Input: part model. Units: mm. Frame: model coordinates. Face numbers are marked on the shaded views. A direction names the side the tool comes from. Round coordinates to 2 decimals unless told otherwise and drop trailing zeros. Write each loop counter-clockwise with the first axis right and the second up, starting at its lowest first coordinate (ties: lowest second). Pieces come first, ordered by that corner, then holes. Notation, with made-up numbers: (82, 11) -> (139, 11) arc R18 cw to (139, 40) -> close; hole circle Ø10 at (63, -25). An arc over 180 degrees is marked (long way). Write item = value, one per line.
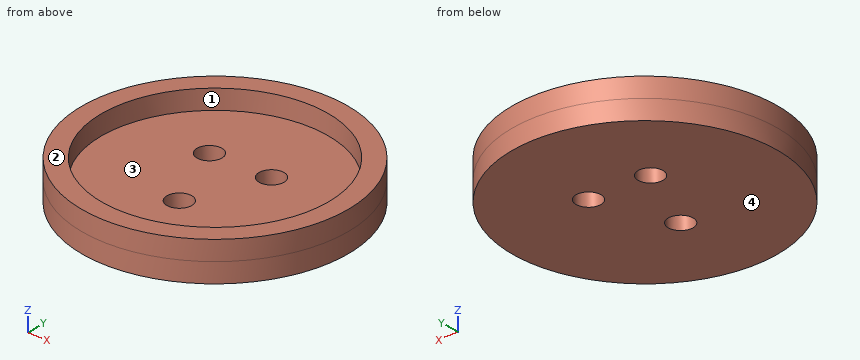
```python
from build123d import *

# Parameters (mm, degrees)
SKETCH1_R      = 24
EXTRUDE1_DEPTH = 4
SKETCH2_R      = 24
EXTRUDE2_DEPTH = 1
SKETCH3_R      = 3.2
EXTRUDE3_DEPTH = 6
SKETCH4_R      = 34
SKETCH4_R_2    = 24
EXTRUDE4_DEPTH = 5
SKETCH5_R      = 34
SKETCH5_R_2    = 29
EXTRUDE5_DEPTH = 5


with BuildPart() as part:
    # Sketch1 → Extrude1 (new body)
    with BuildSketch(Plane.XY):
        Circle(SKETCH1_R)
    extrude(amount=EXTRUDE1_DEPTH)

    # Sketch2 → Extrude2 (add)
    with BuildSketch(Plane.XY.offset(4)):
        Circle(SKETCH2_R)
    extrude(amount=EXTRUDE2_DEPTH)

    # Sketch3 → Extrude3 (cut, through all)
    with BuildSketch(Plane.XY.offset(5)):
        with Locations((-7.9375, 7.9375)):
            Circle(SKETCH3_R)
        with Locations((7.9375, 7.9375)):
            Circle(SKETCH3_R)
        with Locations((0, -11.1125)):
            Circle(SKETCH3_R)
    extrude(amount=-EXTRUDE3_DEPTH, mode=Mode.SUBTRACT)

    # Sketch4 → Extrude4 (add)
    with BuildSketch(Plane(origin=(0, 0, 0), x_dir=(-1, 0, 0), z_dir=(0, 0, -1))):
        Circle(SKETCH4_R)
        Circle(SKETCH4_R_2, mode=Mode.SUBTRACT)
    extrude(amount=-EXTRUDE4_DEPTH)

    # Sketch5 → Extrude5 (add)
    with BuildSketch(Plane.XY.offset(5)):
        Circle(SKETCH5_R)
        Circle(SKETCH5_R_2, mode=Mode.SUBTRACT)
    extrude(amount=EXTRUDE5_DEPTH)


solid = part.part
```
1) Cut plane A-A (x = 0). Return the cut outline in (y, z).
Solutions:
outline = (-34, 0) -> (-14.31, 0) -> (-14.31, 5) -> (-29, 5) -> (-29, 10) -> (-34, 10) -> close; (-7.91, 0) -> (34, 0) -> (34, 10) -> (29, 10) -> (29, 5) -> (-7.91, 5) -> close
2) Draft query along Y for the marked faces 3 and 4. Return one class per face: +Y half, -Y half, draft (parallel to the pull), parting line (faces both ways), or undercut.
Solutions:
face_3 = undercut
face_4 = draft
3) First-contact query: P1, Ø17.5, axis at x = 4.5, y = -2, coming from the +Z side; P2, Ø6, axis at x = 7.94, y = 7.94, coming from the +Z side; P3, Ø6, axis at x = 18, y = 10.5, coming from the -Z side; P4, Ø1.5, axis at y = 3, z = 5.5, coming from the +X side. Flat tips, straight axial feed; report the tip coordinate or a pass-through.
Solutions:
P1 = 5
P2 = through
P3 = 0
P4 = 33.93
4) Access query for the marked faces 1 and 2. Directions: +Z, -Z, +X, -X, +Y, -Y. A direction counts if a zero-diameter tool reaches every point of the face in a straight line with its end or side. Return the directions, or none.
Solutions:
face_1 = +Z
face_2 = +Z, +X, -X, +Y, -Y
5) Cut plane C-C (y = 0). Return the cut outline in (x, z).
Solutions:
outline = (-34, 0) -> (34, 0) -> (34, 10) -> (29, 10) -> (29, 5) -> (-29, 5) -> (-29, 10) -> (-34, 10) -> close
6) Line query: L1, parallel to Y at x = 0, z = 3.2; L2, parallel to Z at x = 8, y = -1.5; L3, parallel to X at y = 9, z = 4. Output: solid intervals per line, ascending. Write a range as from..to.
Solutions:
L1 = -34..-14.31, -7.91..34
L2 = 0..5
L3 = -32.79..-10.96, -4.92..4.92, 10.96..32.79
7) Cut plane B-B (y = 7). Return the cut outline in (x, z).
Solutions:
outline = (-33.27, 0) -> (-11, 0) -> (-11, 5) -> (-28.14, 5) -> (-28.14, 10) -> (-33.27, 10) -> close; (-4.88, 0) -> (4.88, 0) -> (4.88, 5) -> (-4.88, 5) -> close; (11, 0) -> (33.27, 0) -> (33.27, 10) -> (28.14, 10) -> (28.14, 5) -> (11, 5) -> close
8) Cut plane D-D (z = 9). Return the cut outline in (x, y).
Solutions:
outline = circle Ø68 at (0, 0); hole circle Ø58 at (0, 0)
